The model under review builds one solid part; all positions refer to its coordinate system, in mm. A direction names the side the tool comes from. Give positions to 0.01 mm unless a question says otherwise; leave off trailing zeros. Order: outer loops, then holes, each group sorted by start corner. A loop starts at its lowest first (then second) coordinate and runs counter-clockwise, first axis right, second up. Notation, with made-up numbers: (-28.5, 88) - (-20.5, 88) arc R28 cw to (-20.5, 119) - close; hole circle Ø11 at (-10.75, 58). An arc over 180 degrees is marked (long way). Put each result on its own line as item: value.
```python
from build123d import *

# Parameters (mm, degrees)
F1_DEPTH = 400
F2_R     = 25
F3_DEPTH = 600.001


with BuildPart() as f1:
    # F0 (on Front) → F1 (new body)
    with BuildSketch(Plane.XZ):
        Polygon((-150, 300), (-450, 300), (-450, -300), (450, -300), (450, -100), (150, -100), (150, 100), (-150, 100), align=None)
    extrude(amount=F1_DEPTH)

    # F2 (on face) → F3 (cut, through all)
    with BuildSketch(Plane.XY.offset(300)):
        with Locations((-300, -200)):
            Circle(F2_R)
        with Locations((0, -200)):
            Circle(F2_R)
        with Locations((300, -200)):
            Circle(F2_R)
    extrude(amount=-F3_DEPTH, mode=Mode.SUBTRACT)


solid = f1.part
```
(1) Clearance check with flat-ended pins moving along their axes: pin 1 Ø1 at (x, z) = (-246, -205.5) entering from +Y; pin 2 Ø1.5 at (y, z) = (-293.5, -49.5) entering from +X. State where each tip first meets the part, or that it passes through.
The answers:
pin 1: y = 0
pin 2: x = 150
(2) Take a section at A-A, the plane x = -300. Write out the cut boundary in (y, z), then the cut area to 3 significant figures.
The answers:
outline: (-400, -300) - (-225, -300) - (-225, 300) - (-400, 300) - close; (-175, -300) - (0, -300) - (0, 300) - (-175, 300) - close
area: 210,000 mm^2
(3) Take a section at C-C, the plane z = 54.5. Write out the cut boundary in (x, y).
The answers:
outline: (-450, -400) - (150, -400) - (150, 0) - (-450, 0) - close; hole circle Ø50 at (-300, -200); hole circle Ø50 at (0, -200)
(4) Wall thickness on L1, parallel to Y at x = 300, z = -180; L2, parallel to Z at x = 244.5, y = -90; L3, parallel to Z at x = 35.5, y = -267: over which ranges is each line inside the solid? List them lowest first.
The answers:
L1: -400 to -225, -175 to 0
L2: -300 to -100
L3: -300 to 100
(5) The part is to be moulded in two halves that separate along Y. For faces 3 (the cylindrical face through (-3.255, -175.213, -97.2)), 4 (the flat face through (-450, -197, 4)), 5 (the flat face through (-106, -400, -62)), 6 (the flat face through (-106, 0, -62)), say which applies: pulls with the +Y half, pulls with the -Y half, needs draft (parallel to the pull), parting line crosses it, or undercut.
The answers:
face 3: undercut
face 4: needs draft
face 5: pulls with the -Y half
face 6: pulls with the +Y half
(6) Take a section at B-B, the plane y = -200. Write out the cut boundary in (x, z).
The answers:
outline: (-450, -300) - (-325, -300) - (-325, 300) - (-450, 300) - close; (-275, -300) - (-25, -300) - (-25, 100) - (-150, 100) - (-150, 300) - (-275, 300) - close; (25, -300) - (275, -300) - (275, -100) - (150, -100) - (150, 100) - (25, 100) - close; (325, -300) - (450, -300) - (450, -100) - (325, -100) - close
(7) Take a section at D-D, the plane y = -88.5. Write out the cut boundary in (x, z).
The answers:
outline: (-450, -300) - (450, -300) - (450, -100) - (150, -100) - (150, 100) - (-150, 100) - (-150, 300) - (-450, 300) - close
(8) For faces 1 (the cylindrical face through (323.846, -192.491, -198.6)), 2 (the flat face through (269, -197, -100)), list the 3-axis set-ups (+Z, -Z, +X, -X, +Y, -Y) from which the entire face can be reached by the end or side of a thin tool; tool diameter is ignored.
The answers:
face 1: +Z, -Z
face 2: +Z, +X, +Y, -Y
